```python
from build123d import *

# Parameters (mm, degrees)
BOSS_EXTRUDE1_DEPTH                                 = 914.4
CUT_EXTRUDE1_REACH                                  = 918.888
SKETCH2_R                                           = 43.18
CUT_EXTRUDE2_DEPTH                                  = 1219.2
CSK_FOR_3_8_FLAT_HEAD_MACHINE_SCREW_100_D           = 10.0838
CSK_FOR_3_8_FLAT_HEAD_MACHINE_SCREW_100_CSINK_D     = 19.3548
CSK_FOR_3_8_FLAT_HEAD_MACHINE_SCREW_100_CSINK_ANGLE = 100


with BuildPart() as part:
    # Sketch1 → Boss-Extrude1 (new body)
    with BuildSketch(Plane.XY):
        Polygon((0, 50.8), (0, 0), (50.8, 0), (50.8, 6.35), (6.35, 6.35), (6.35, 50.8), align=None)
    extrude(amount=BOSS_EXTRUDE1_DEPTH)

    # Sketch2 → Cut-Extrude1 (cut, up to next)
    with BuildSketch(Plane(origin=(0, 6.35, 0), x_dir=(1, 0, 0), z_dir=(0, 1, 0)), mode=Mode.PRIVATE) as cut_extrude1_sk1:
        with Locations((25.4, 0)):
            Circle(SKETCH2_R)
    cut_extrude1_tool1 = extrude(cut_extrude1_sk1.sketch, amount=CUT_EXTRUDE1_REACH, mode=Mode.PRIVATE) & part.part
    add(cut_extrude1_tool1.solids().sort_by_distance((25.4, 6.35, 0))[0], mode=Mode.SUBTRACT)

    # Sketch3 → Cut-Extrude2 (cut)
    with BuildSketch(Plane(origin=(0, 6.35, 0), x_dir=(1, 0, 0), z_dir=(0, 1, 0))):
        with BuildLine():
            Line((25.4, 0), (-1.540768363, -26.940768363))
            ThreePointArc((-1.540768363, -26.940768363), (25.4, 38.1), (52.340768363, -26.940768363))
            Line((52.340768363, -26.940768363), (25.4, 0))
        make_face()
    extrude(amount=-CUT_EXTRUDE2_DEPTH, mode=Mode.SUBTRACT)

    # CSK for 3/8 Flat Head Machine Screw (100)1 (through all)
    with Locations(Plane(origin=(0, 0, 0), x_dir=(-1, 0, 0), z_dir=(0, -1, 0))):
        with Locations((-25.4, -19.05)):
            CounterSinkHole(CSK_FOR_3_8_FLAT_HEAD_MACHINE_SCREW_100_D / 2, CSK_FOR_3_8_FLAT_HEAD_MACHINE_SCREW_100_CSINK_D / 2, counter_sink_angle=CSK_FOR_3_8_FLAT_HEAD_MACHINE_SCREW_100_CSINK_ANGLE)


solid = part.part
```
Input: part model. Units: mm. Frame: model coordinates. A direction names the side the tool comes from. Coordinates: 2 decimals unless noted, no trailing zeros. Loops run counter-clockwise (first coordinate to the right, second up) from the corner with the lowest first, then second, coordinate; pieces in that order, holes last. Notation, with made-up numbers: (-26, 63) -> (14, 63) arc R27 cw to (14, 81) -> close; hole circle Ø5 at (1, 82). An arc over 180 degrees is marked (long way). Use a Markdown table: item, result.
1) Contact query for flat-ended pins moving along their axis: pin 1 (3 mm diameter, centred on x = 40, z = 201, fed in from +Y); pin 2 (10 mm diameter, centred on x = 6.5, z = 559.5, fed in from +Y); pin 3 (12 mm diameter, centred on x = 39.5, y = 10, fed in from -Z); pin 4 (11.5 mm diameter, centred on x = 25.4, z = 19.05, fed in from -Y). Output: stop coordinate, or through.
Results found:
| item | result |
|---|---|
| pin 1 | stops at y = 6.35 |
| pin 2 | stops at y = 50.8 |
| pin 3 | stops at z = 9.34 |
| pin 4 | stops at y = 3.3 |
2) Pull-direction query (Z, two-part tool) for faces 3 (the conical face through (20.14, 3.7, 18.82)), 4 (the flat face through (12.9, 3.2, 12.5)), 5 (the flat face through (0, 26, 464)); classes: released by +Z, released by -Z, zero draft, split by the parting line, or undercut.
Results found:
| item | result |
|---|---|
| face 3 | undercut |
| face 4 | released by -Z |
| face 5 | zero draft |
3) Cut plane A-A (y = 30). Return the cut outline in (x, z).
Results found:
| item | result |
|---|---|
| outline | (0, 34.92) arc R43.18 cw to (6.35, 38.75) -> (6.35, 914.4) -> (0, 914.4) -> close |
4) Cut plane B-B (z = 521). Return the cut outline in (x, y).
Results found:
| item | result |
|---|---|
| outline | (0, 0) -> (50.8, 0) -> (50.8, 6.35) -> (6.35, 6.35) -> (6.35, 50.8) -> (0, 50.8) -> close |
5) Access query for faces 1 (the flat face through (14, 5, 914.4)), 2 (the flat face through (6.35, 28, 470)). Directions: +Z, -Z, +X, -X, +Y, -Y. A direction counts if a zero-diameter tool reaches every point of the face in a straight line with its end or side. Return the directions, or none.
Results found:
| item | result |
|---|---|
| face 1 | +Z, +X, -X, +Y, -Y |
| face 2 | +Z, -Z, +X, +Y |
6) Material intervals for line 1 along Z through (x, y) = (25.4, 5.1); line 2 along Y through (x, z) = (38, 644); line 3 along Z through (x, y) = (25, 5), sorted ascending. Write a range as from..to.
Results found:
| item | result |
|---|---|
| line 1 | z = 0..14.01, 24.09..914.4 |
| line 2 | y = 0..6.35 |
| line 3 | z = 0.4..14.02, 24.08..914.4 |
